Design review of the part built by this model. Coordinates are the model's own, in mm. A direction names the side the tool comes from. Round coordinates to 2 decimals unless told otherwise and drop trailing zeros. Write each loop counter-clockwise with the first axis right and the second up, starting at its lowest first coordinate (ties: lowest second). Pieces come first, ordered by that corner, then holes. Notation, with made-up numbers: (63.5, -34.75) - (109.5, -34.75) arc R15 ccw to (109.5, -29.75) - close; hole circle Ø6 at (41.25, 19). An arc over 180 degrees is marked (long way). Use one line per item in the form item = value.
Autodesk Inventor part; units mm, degrees
ref_plane "Arbeitsebene1" through (0, 9, 0) normal (0, 1, 0) x (-1, 0, 0)
ref_plane "YZ Plane" through (0, 0, 0) normal (1, 0, 0) x (0, 1, 0)
ref_plane "XY Plane" through (0, 0, 0) normal (0, 0, 1) x (1, 0, 0)
sketch "Skizze4" plane through (0, 0, 0) normal (0, 0, 1) x (1, 0, 0)
  line L0 (-12.6, 0) -> (12.6, 0)
  line L1 (0, -12.6) -> (0, 12.6)
  circle A0 centre (0, 0) radius 9
  point P0 (-9, 0)
  point P1 (9, 0)
  dimension "d8" = 18
revolve "Umdrehung1" add sketch "Skizze4" angle 360 about axis through (-10, 0, 0) along (1, 0, 0) picked at (-5.0484, 3.1721) picked at (5.9248, 0.6676) contours A0 L1 L0 | L1 A0 L0
ref_plane "Arbeitsebene1" through (0, 9, 0) normal (0, 1, 0) x (-1, 0, 0)
sketch "Skizze5" plane through (0, 9, 0) normal (0, 1, 0) x (-1, 0, 0)
  circle A0 centre (0, 0) radius 2.5
  dimension "d11" = 5
extrude "Extrusion3" add sketch "Skizze5" along normal mid plane 1
sketch "Skizze6" plane through (0, 9.5, 0) normal (0, 1, 0) x (1, 0, 0)
  circle A0 centre (0, 0) radius 2.5
  circle A1 centre (0, 0) radius 2.5
  dimension "d14" = 5
extrude "Extrusion4" add sketch "Skizze6" along normal blind 2
sketch "Skizze7" plane through (0, 0, 0) normal (0, 0, 1) x (1, 0, 0)
  circle A0 centre (0, 0) radius 5
  dimension "d17" = 10
extrude "Extrusion5" cut sketch "Skizze7" along normal mid plane 20
sketch "Skizze8" plane through (0, 11.5, 0) normal (0, 1, 0) x (1, 0, 0)
  circle A0 centre (0, 0) radius 7.9569
  dimension "d20" = 15.9138
extrude "Extrusion6" add sketch "Skizze8" along normal blind 5
sketch "Skizze9" plane through (0, 0, 0) normal (1, 0, 0) x (0, 1, 0)
  line L0 (16.5, -7.9569) -> (16.5, 7.9569)
  line L1 (11.5, -7.9569) -> (11.5, 7.9569)
  line L2 (16.5, 7.9569) -> (11.5, 7.9569)
  line L3 (11.5, 7.9569) -> (11.5, -7.9569)
  line L4 (11.5, -7.9569) -> (16.5, -7.9569)
  line L5 (16.5, -7.9569) -> (16.5, 7.9569)
  point P0 (0, 0)
extrude "Extrusion7" add sketch "Skizze9" along normal blind 10
sketch "Skizze10" plane through (0, 16.5, 0) normal (0, 1, 0) x (1, 0, 0)
  line L0 (10, 7.9569) -> (10, -7.9569)
  line L1 (0, 7.9569) -> (10, 7.9569)
  line L2 (10, -7.9569) -> (5, -7.9569)
  line L3 (5, -7.9569) -> (5, 7.9569)
  line L4 (5, 7.9569) -> (10, 7.9569)
  line L5 (10, 7.9569) -> (10, -7.9569)
  point P0 (0, 0)
  dimension "d25" = 5
extrude "Extrusion8" add sketch "Skizze10" along normal blind 5
sketch "Skizze11" plane through (10, 0, 0) normal (1, 0, 0) x (0, 0, -1)
  line L0 (7.9569, 11.5) -> (7.9569, 21.5)
  line L1 (-7.9569, 11.5) -> (-7.9569, 21.5)
  line L2 (7.9569, 21.5) -> (-7.9569, 21.5)
  line L3 (-7.9569, 21.5) -> (-7.9569, 16.5)
  line L4 (-7.9569, 16.5) -> (7.9569, 16.5)
  line L5 (7.9569, 16.5) -> (7.9569, 21.5)
  point P0 (0, 0)
  point P1 (7.9569, 16.5)
  dimension "d28" = 5
extrude "Extrusion9" add sketch "Skizze11" along normal blind 80
fillet "Rundung2" radius 2 2 edges at (10, 11.5, 0) (5, 21.5, 0)
fillet "Rundung3" radius 5 2 edges at (90, 19, 7.9569) (90, 19, -7.9569)
sketch "Skizze12" plane through (0, 21.5, 0) normal (0, 1, 0) x (1, 0, 0)
  circle A0 centre (85, 0) radius 1.5
  line L0 (90, 2.9569) -> (90, -2.9569)
  point P0 (0, 0)
  dimension "d33" = 3
  dimension "d34" = 5
extrude "Extrusion10" cut sketch "Skizze12" against normal blind 5
properties part number "VentilNukleator2"
Q1. We need section C-C on x = 76.5. Write out the cut boundary in (y, z), then the cut area to 3 significant figures.
Calculated:
outline = (16.5, -7.96) - (21.5, -7.96) - (21.5, 7.96) - (16.5, 7.96) - close
area = 79.6 mm2
Q2. We need section B-B on y = 0. Write out the cut boundary in (x, z), then the cut area to 3 significant figures.
Calculated:
outline = (-5, -7.48) - (-5, 7.48) arc R9 ccw to start; (5, -7.48) arc R9 ccw to (5, 7.48) - close
area = 84.2 mm2
Q3. Draft analysis for pull direction Z (two halves, no side actions). For faces 1 (the cylindrical face through (86.43, 19.04, -0.45)), 2 (the flat face through (42, 19, -7.957)), 3 (the flat face through (42, 19, 7.957)), state which applies: released by +Z, released by -Z, zero draft, split by the parting line, or undercut.
Calculated:
face_1 = undercut
face_2 = released by -Z
face_3 = released by +Z
Q4. To check wall thickness, follow line 1 along Z through (x, y) = (85, 19.25); line 2 along X through (y, z) = (19.4, 0); line 3 along Y through (x, z) = (0, -3.75). State the ranges of each line that lie inside material, in increasing order. Write a range as from..to.
Calculated:
line_1 = -7.96..-1.5, 1.5..7.96
line_2 = 5..83.5, 86.5..90
line_3 = -8.18..-5, 5..8.18, 11.5..16.5
Q5. Machinability: for faces 4 (the cylindrical face through (9.4, 12.07, 0.11)), 5 (the flat face through (49, 16.5, 0)), 6 (the flat face through (5, 18, 0)), 7 (the flat face through (2, 11.5, -2)), which of the approach directions +Z, -Z, +X, -X, +Y, -Y give a long, thin tool a straight path to every point of the face, cutting with its end or side? Answer none if there is none.
Calculated:
face_4 = +Z, -Z, +X
face_5 = +Z, -Z, +X, -Y
face_6 = +Z, -Z, -X, +Y
face_7 = none
Q6. For P1, Ø13, axis at x = 0, y = 0, coming from the +Z side; P2, Ø5, axis at y = 13, z = 1.5, coming from the +X side; P3, Ø0.9, axis at y = 18, z = -4, coming from the -X side; P4, Ø2.5, axis at y = 15.5, z = 2.5, coming from the +X side, all flat-tipped, find the tip position at first contact; note any pin that passes through.
Calculated:
P1 = 7.48
P2 = 10
P3 = 5
P4 = 90
Q7. We need section A-A on z = 4.5. Write out the cut boundary in (x, y).
Calculated:
outline = circle Ø15.59 at (0, 0); (-6.56, 11.5) - (8, 11.5) arc R2 ccw to (10, 13.5) - (10, 16.5) - (89.76, 16.5) - (89.76, 21.5) - (7, 21.5) arc R2 ccw to (5, 19.5) - (5, 16.5) - (-6.56, 16.5) - close; hole circle Ø10 at (0, 0)
